Study the drawing (mm; zero at the part's minimum x, y, z) and answer. Round coordinates to 2 decimals unless told otherwise and drop trailing zeros. Order: outer loops, then holes, each group sorted by start corner. A loop starts at its lowest first (then second) coordinate and runs counter-clockwise, first axis right, second up. Notation, with made-up numbers: (47, 78) - (105, 78) arc R5 cw to (105, 82) - close; hole circle Ø9 at (2.5, 56). An arc over 180 degrees is marked (long way). Use one line per item in the form item = value. Start each with the question number.
Q1. The part is cut by section C-C on z = 12.75. Determine the outline of the cut face in (x, y).
Q2. Find the intervals of material crossed by line 1 (Z direction, x = 9.75, y = 143.5); line 2 (Z direction, x = 8, y = 81); line 3 (X direction, y = 7.5, z = 14.75), in increasing order. Write a range as [from, to].
Q3. The part is cut by section A-A on y = 56. Determine the outline of the cut face in (x, z), plus the area to 3 significant figures.
Q4. Given P1, Ø5, axis at x = 14, y = 39.5, coming from the -Z side; P2, Ø5, axis at y = 87, z = 2, coming from the -X side, each flat-ended and moving along its own axis, determine where each tip first touches the part or whether it passes through.
Q5. The part is cut by section B-B on x = 2. Determine the outline of the cut face in (y, z).
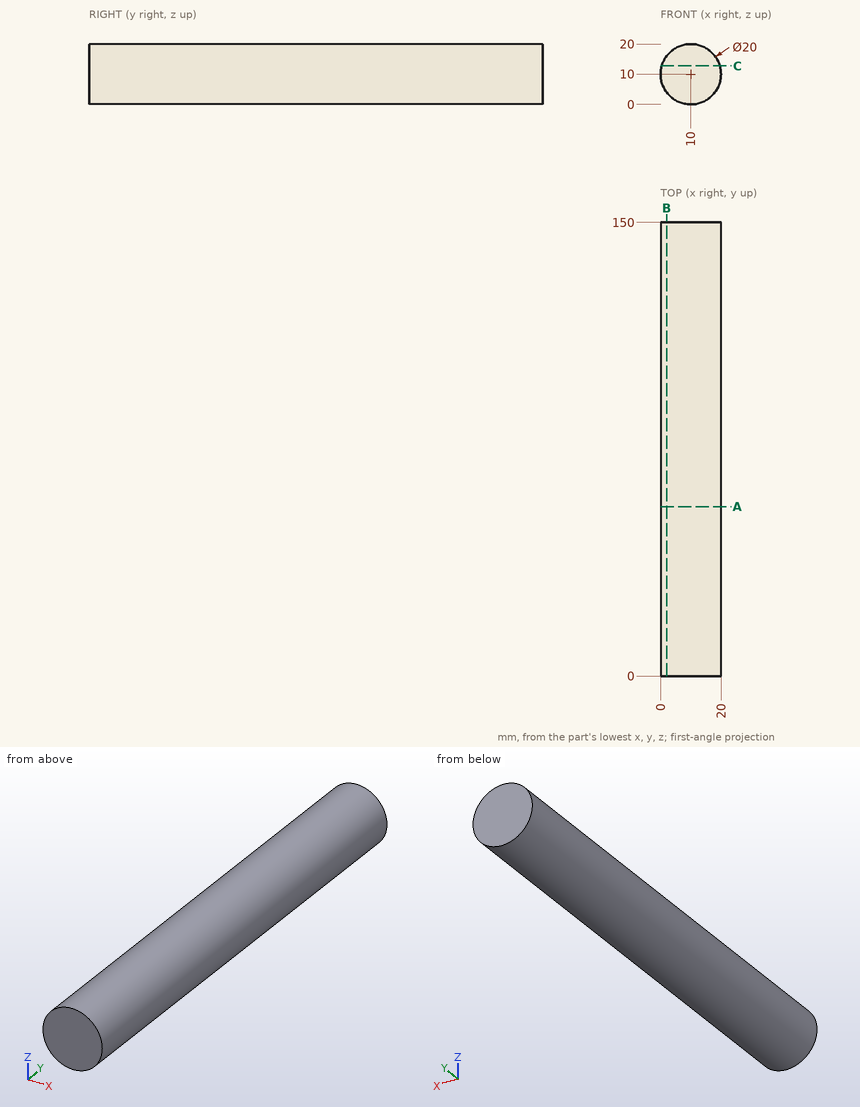
Found:
q1.outline = (0.39, 0) - (19.61, 0) - (19.61, 150) - (0.39, 150) - close
q2.line_1 = [0, 20]
q2.line_2 = [0.2, 19.8]
q2.line_3 = [1.2, 18.8]
q3.outline = circle Ø20 at (10, 10)
q3.area = 314 mm²
q4.P1 = 0.11
q4.P2 = 1.65
q5.outline = (0, 4) - (150, 4) - (150, 16) - (0, 16) - close
